Could you check a few things on this model? Use its own coordinates, in mm. Face numbers are marked on the shaded views. A direction names the side the tool comes from. Give positions to 0.01 mm unless a question says otherwise; leave off trailing zeros. Order: outer loops, then holes, each group sorted by start corner. A loop starts at its lowest first (then second) coordinate and runs counter-clockwise, first axis right, second up. Notation, with made-up numbers: M 65.5,43 L 81.5,43 A5 ccw 81.5,49 Z; hole C 11,-9 d2. An arc over 180 degrees is marked long. Use a Markdown table: item, result. Add a question column.
Item 1: If we mould it in two halves opening along X, with no side actions, what happens to the marked faces 1, 2 and 3? For each: released by +X, released by -X, zero draft, split by the parting line, or undercut.
Item 2: For the marked faces 4 and 5, which set-ups out of +Z, -Z, +X, -X, +Y, -Y let a thin tool reach every point of the face, with its end or its side?
Item 3: If I drill on L1, parallel to Y at x = 0, z = 3.5; L2, parallel to Y at x = 1.75, z = -4; L3, parallel to X at y = 4, z = 2, over which ranges is the centre line in solid material (lowest first)? Write a range as from..to.
Item 4: Suppose I cut it at A-A on z = 7.25. Write out the boundary of the cut face in (x, y).
Item 5: Suppose I cut it at B-B on y = 6. Write out the boundary of the cut face in (x, z), plus the area to 4 significant figures.
Item 6: I'm going to push a flat-ended pin straight in: pin 1 Ø1.5 at (x, z) = (1, -6.5) entering from +Y. Where does the tip first touch, or does it pass through?
Item 7: Suppose I cut it at C-C on x = 4.75. Write out the boundary of the cut face in (y, z).
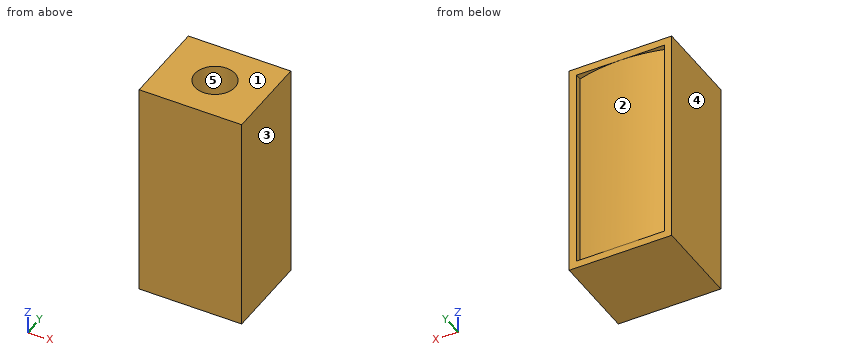
Autodesk Inventor part; units mm, degrees
ref_plane "YZ Plane" through (0, 0, 0) normal (1, 0, 0) x (0, 1, 0)
ref_plane "XZ Plane" through (0, 0, 0) normal (0, 1, 0) x (-1, 0, 0)
ref_plane "XY Plane" through (0, 0, 0) normal (0, 0, 1) x (1, 0, 0)
sketch "Sketch1" plane through (0, 0, 0) normal (0, 1, 0) x (-1, 0, 0)
  line L0 (-7, 15) -> (-7, -15)
  line L1 (-7, -15) -> (7, -15)
  line L2 (7, -15) -> (7, 15)
  line L3 (7, 15) -> (-7, 15)
  line L4 (-7, 15) -> (7, -15) construction
  line L5 (-7, -15) -> (7, 15) construction
  point P0 (0, 0)
  dimension "d0" = 30
  dimension "d1" = 14
extrude "Extrusion1" add sketch "Sketch1" along normal blind 12
sketch "Sketch2" plane through (-7, 0, 15) normal (0, 0, 1) x (1, 0, 0)
  circle A0 centre (7, 6) radius 2.75
  point P0 (7, 0)
  dimension "d4" = 5.5
extrude "Extrusion2" cut sketch "Sketch2" against normal blind 25
sketch "Sketch3" plane through (0, 12, 0) normal (0, 1, 0) x (1, 0, 0)
  line L0 (7, -15) -> (7, 15)
  line L1 (7, 15) -> (-7, 15)
  line L2 (-7, 15) -> (-7, -15)
  line L3 (-7, -15) -> (7, -15)
  line L4 (-6, -14) -> (-6, 14)
  line L5 (-6, 14) -> (6, 14)
  line L6 (6, 14) -> (6, -14)
  line L7 (6, -14) -> (-6, -14)
  point P0 (0, 0)
  dimension "d7" = 1
sketch "Sketch4" plane through (0, 0, 0) normal (0, 0, 1) x (1, 0, 0)
  line L0 (7, 12) -> (-7, 12)
  line L1 (-7, 12) -> (7, 0)
  line L2 (7, 0) -> (7, 12)
  line L3 (7, 0) -> (7, 12)
  line L4 (7, 12) -> (-7, 0)
  line L5 (-7, 0) -> (-6, 0)
  line L6 (7, 0) -> (-7, 0)
  line L7 (-6, 0) -> (-6, 12)
  arc A0 (5.9979, 11.1411) -> (-6, 11.1429) centre (-0.0041, -9.3998) ccw
  line L8 (5.9979, 11.1411) -> (5.9979, 12)
  point P0 (0, 0)
  dimension "d8" = 1
extrude "Extrusion3" cut sketch "Sketch4" along normal mid plane 28 contours L8 A0 L0 | A0 L7 L0
properties part number "Solonoid Outside"
Findings below:
| question | item | result |
|---|---|---|
| 1 | face 1 | zero draft |
| 1 | face 2 | undercut |
| 1 | face 3 | released by +X |
| 2 | face 4 | +Z, -Z, -X, +Y, -Y |
| 2 | face 5 | +Z |
| 3 | L1 | y = 0..3.25, 8.75..12 |
| 3 | L2 | y = 0..3.88, 8.12..11.93 |
| 3 | L3 | x = -7..-1.89, 1.89..7 |
| 4 | outline | M -7,0 L 7,0 L 7,12 L 6,12 L 6,11.14 A21.4 ccw -6,11.14 L -6,12 L -7,12 Z; hole C 0,6 d5.5 |
| 5 | outline | M -7,-15 L 7,-15 L 7,15 L 2.75,15 L 2.75,-10 L -2.75,-10 L -2.75,15 L -7,15 Z |
| 5 | area | 282.5 mm^2 |
| 6 | pin 1 | stops at y = 12 |
| 7 | outline | M 0,-15 L 12,-15 L 12,-14 L 11.47,-14 L 11.47,14 L 12,14 L 12,15 L 0,15 Z |
